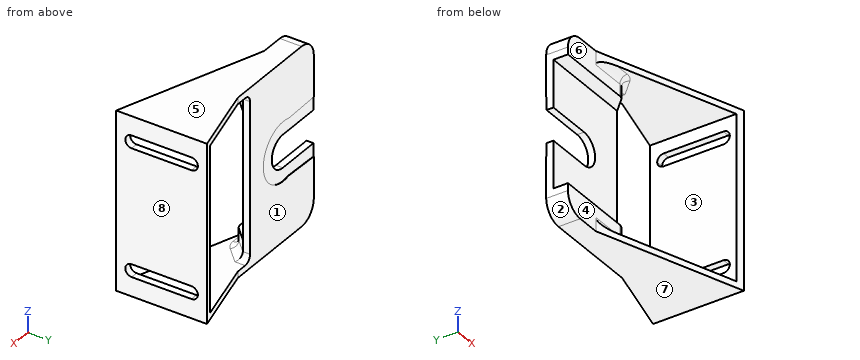
from build123d import *

# Parameters (mm, degrees)
F1_DEPTH  = 49
F3_DEPTH  = 8.001
F4_W      = 18
F4_H      = 45.5
F4_W_2    = 5
F5_DEPTH  = 25
F7_DEPTH  = 2
F8_W      = 33.7460841984
F8_H      = 45.5
F9_DEPTH  = 18.001
F11_DEPTH = 0.1
F12_W     = 26
F12_H     = 1.75
F12_H_2   = 5.25
F13_DEPTH = 4
F14_SIZE  = 4
F15_R     = 2
F16_R     = 5


# Not quite as in the source:
# - a feature names something its author has since deleted; it is built from what else it names


with BuildPart() as f1:
    # F0 (on Top) → F1 (new body)
    with BuildSketch(Plane.XY):
        Polygon((31, 2), (0, 2), (0, 0), (51, -18), (51, 2), align=None)
        Polygon((51, 7), (31, 2), (51, 2), align=None)
    extrude(amount=F1_DEPTH)

    # F2 (on face) → F3 (cut, through all)
    with BuildSketch(Plane(origin=(0, 2, 0), x_dir=(-1, 0, 0), z_dir=(0, 1, 0))):
        with BuildLine():
            Line((0, 29), (-12.5, 29))
            ThreePointArc((-12.5, 29), (-17, 24.5), (-12.5, 20))
            Line((-12.5, 20), (0, 20))
            Line((0, 20), (0, 29))
        make_face()
    extrude(amount=-F3_DEPTH, mode=Mode.SUBTRACT)

    # F4 (on face) → F5 (cut, symmetric)
    with BuildSketch(Plane(origin=(0, 2, 0), x_dir=(-1, 0, 0), z_dir=(0, 1, 0))):
        with Locations((-40, 24.5)):
            Rectangle(F4_W, F4_H)
        with Locations((-28.5, 24.5)):
            Rectangle(F4_W_2, F4_H)
    extrude(amount=F5_DEPTH, both=True, mode=Mode.SUBTRACT)

    # F6 (on face) → F7 (cut, through all)
    with BuildSketch(Plane.YZ.offset(51)):
        with BuildLine():
            ThreePointArc((2.75, 40.25), (1, 42), (2.75, 43.75))
            Line((2.75, 43.75), (-13.75, 43.75))
            ThreePointArc((-13.75, 43.75), (-12.5125631329, 43.2374368671), (-12, 42))
            ThreePointArc((-12, 42), (-12.5125631329, 40.7625631329), (-13.75, 40.25))
            Line((-13.75, 40.25), (2.75, 40.25))
        make_face()
        with BuildLine():
            ThreePointArc((-12, 42), (-12.5125631329, 43.2374368671), (-13.75, 43.75))
            ThreePointArc((-13.75, 43.75), (-15.5, 42), (-13.75, 40.25))
            ThreePointArc((-13.75, 40.25), (-12.5125631329, 40.7625631329), (-12, 42))
        make_face()
        with BuildLine():
            ThreePointArc((2.75, 40.25), (3.9874368671, 40.7625631329), (4.5, 42))
            ThreePointArc((4.5, 42), (3.9874368671, 43.2374368671), (2.75, 43.75))
            ThreePointArc((2.75, 43.75), (1, 42), (2.75, 40.25))
        make_face()
        with BuildLine():
            ThreePointArc((2.75, 5.25), (1, 7), (2.75, 8.75))
            Line((2.75, 8.75), (-13.75, 8.75))
            ThreePointArc((-13.75, 8.75), (-12.5125631329, 8.2374368671), (-12, 7))
            ThreePointArc((-12, 7), (-12.5125631329, 5.7625631329), (-13.75, 5.25))
            Line((-13.75, 5.25), (2.75, 5.25))
        make_face()
        with BuildLine():
            ThreePointArc((-12, 7), (-12.5125631329, 8.2374368671), (-13.75, 8.75))
            ThreePointArc((-13.75, 8.75), (-15.5, 7), (-13.75, 5.25))
            ThreePointArc((-13.75, 5.25), (-12.5125631329, 5.7625631329), (-12, 7))
        make_face()
        with BuildLine():
            ThreePointArc((4.5, 7), (3.9874368671, 8.2374368671), (2.75, 8.75))
            ThreePointArc((2.75, 8.75), (1, 7), (2.75, 5.25))
            ThreePointArc((2.75, 5.25), (3.9874368671, 5.7625631329), (4.5, 7))
        make_face()
    extrude(amount=-F7_DEPTH, mode=Mode.SUBTRACT)

    # F8 (on Front) → F9 (cut, through all)
    with BuildSketch(Plane.XZ):
        with Locations((14.1801619902, 24.5)):
            Rectangle(F8_W, F8_H)
    extrude(amount=F9_DEPTH, mode=Mode.SUBTRACT)

    # F10 (on face) → F11 (cut)
    with BuildSketch(Plane(origin=(0, 2, 0), x_dir=(-1, 0, 0), z_dir=(0, 1, 0))):
        with BuildLine():
            ThreePointArc((-10.3159670332, 16.7), (-6.0462930408, 19.6051387676), (-4.4, 24.5))
            ThreePointArc((-4.4, 24.5), (-6.0462930408, 29.3948612324), (-10.3159670332, 32.3))
            ThreePointArc((-10.3159670332, 32.3), (-20.6, 24.5), (-10.3159670332, 16.7))
        make_face()
        with BuildLine():
            ThreePointArc((-10.3159670332, 32.3), (-6.0462930408, 29.3948612324), (-4.4, 24.5))
            ThreePointArc((-4.4, 24.5), (-6.0462930408, 19.6051387676), (-10.3159670332, 16.7))
            Line((-10.3159670332, 16.7), (0, 16.4))
            Line((0, 16.4), (0, 32.6))
            Line((0, 32.6), (-10.3159670332, 32.3))
        make_face()
    extrude(amount=-F11_DEPTH, mode=Mode.SUBTRACT)

    # F12 (on face) → F13 (join)
    with BuildSketch(Plane.XZ):
        with Locations((13, 48.125)):
            Rectangle(F12_W, F12_H)
        with Locations((13, 0.875)):
            Rectangle(F12_W, F12_H)
        with Locations((13, 44.625)):
            Rectangle(F12_W, F12_H_2)
        with Locations((13, 4.375)):
            Rectangle(F12_W, F12_H_2)
    extrude(amount=F13_DEPTH)

    # F14
    f14_edges = [f1.edges().sort_by_distance(p)[0] for p in [
        (26, -4, 4.375),
        (26, -4, 44.625),
    ]]
    chamfer(f14_edges, length=F14_SIZE)

    # F15
    f15_edges = [f1.edges().sort_by_distance(p)[0] for p in [
        (16.666667, -4, 1.75),
        (16.666667, -4, 47.25),
        (24, -2, 47.25),
        (24, -2, 1.75),
        (22, -4, 4.375),
        (22, -4, 44.625),
        (26, 1, 1.75),
        (26, 1, 47.25),
    ]]
    fillet(f15_edges, radius=F15_R)

    # F16
    f16_edges = [f1.edges().sort_by_distance(p)[0] for p in [
        (0, -1, 49),
        (0, -1, 0),
    ]]
    fillet(f16_edges, radius=F16_R)


solid = f1.part
Design review of the part built by this model. Coordinates are the model's own, in mm. Face numbers are marked on the shaded views. A direction names the side the tool comes from. Round coordinates to 2 decimals unless told otherwise and drop trailing zeros. Loops run counter-clockwise (first coordinate to the right, second up) from the corner with the lowest first, then second, coordinate; pieces in that order, holes last. Notation, with made-up numbers: (-6.5, 20) -> (2.5, 20) arc R24 cw to (2.5, 50) -> close; hole circle Ø11 at (-34.5, -19). An arc over 180 degrees is marked (long way). Use one line per item in the form item = value. Start each with the question number.
Q1. We need section C-C on x = 37. Give the boundary of the cut face in (y, z), then the cut area to 3 significant figures.
Q2. Machinability: for the marked faces 1, 2, 3, 4 and 5, which of the approach directions +Z, -Z, +X, -X, +Y, -Y give a long, thin tool a straight path to every point of the face, cutting with its end or side? Answer none if there is none.
Q3. Wall thickness on line 1 along Z through (x, y) = (26, -5.75); line 2 along Y through (x, z) = (12, 39); line 3 along X through (y, z) = (2.05, 24.5): over which ranges is each line inside the solid? List them lowest first. Write a range as [from, to].
Q4. We need section D-D on y = -2.25. State how many separate pieces and enclosed holes the cut face has, then the cut area to 3 significant figures.
Q5. We need section A-A on z = 24.5. Give the boundary of the cut face in (x, y), then the cut area to 3 significant figures.
Q6. Draft analysis for pull direction Z (two halves, no side actions). For the marked faces 6, 7 and 8, state which applies: +Z half, -Z half, draft (parallel to the pull), parting line (faces both ways), or undercut.
Q7. For pin 1 Ø2 at (x, z) = (20, 6.5) entering from -Y; pin 2 Ø1 at (y, z) = (-4, 31) entering from -X; pin 3 Ø18 at (x, z) = (7, 22) entering from +Y, all flat-tipped, find the tip position at first contact; note any pin that passes through.
Q8. We need section B-B on y = -12. Give the boundary of the cut face in (x, z).
Calculated:
q1.outline = (-13.06, 0) -> (3.5, 0) -> (3.5, 1.75) -> (-13.06, 1.75) -> close; (-13.06, 47.25) -> (3.5, 47.25) -> (3.5, 49) -> (-13.06, 49) -> close
q1.area = 58.0 mm²
q2.face_1 = +Z, -Z, -X, +Y
q2.face_2 = -Z, -X, +Y, -Y
q2.face_3 = +Y, -Y
q2.face_4 = -X, -Y
q2.face_5 = +Z, +X, -X, +Y, -Y
q3.line_1 = [0, 1.75], [47.25, 49]
q3.line_2 = [0, 2]
q3.line_3 = [49, 51]
q4.separate_pieces = 3
q4.enclosed_holes = 0
q4.area = 497 mm²
q5.outline = (17, 0) -> (26, 0) -> (26, 2) -> (20.6, 2) -> (20.6, 1.9) -> (17, 1.9) -> close; (49, -17.29) -> (51, -18) -> (51, 7) -> (49, 6.5) -> close
q5.area = 66.4 mm²
q6.face_6 = undercut
q6.face_7 = -Z half
q6.face_8 = draft
q7.pin_1 = -4
q7.pin_2 = 49
q7.pin_3 = 2
q8.outline = (34, 0) -> (51, 0) -> (51, 5.25) -> (49, 5.25) -> (49, 1.75) -> (34, 1.75) -> close; (34, 47.25) -> (49, 47.25) -> (49, 43.75) -> (51, 43.75) -> (51, 49) -> (34, 49) -> close; (49, 8.75) -> (51, 8.75) -> (51, 40.25) -> (49, 40.25) -> close
